from build123d import *

# Parameters (mm, degrees)
CUT_EXTRUDE1_DEPTH      = 10
BOSS_EXTRUDE1_DEPTH     = 30
CUT_EXTRUDE2_DEPTH      = 752.943114111524
CUT_EXTRUDE2_DEPTH_BACK = 752.943114111524
SKETCH5_R               = 4.999999999999998
SKETCH6_R               = 40.00000000000003
CUT_EXTRUDE3_DEPTH      = 752.943114111524
BOSS_EXTRUDE3_DEPTH     = 5
CUT_EXTRUDE4_DEPTH      = 752.943114111524
CUT_EXTRUDE4_DEPTH_BACK = 752.943114111524
FILLET1_R               = 5
FILLET2_R               = 4.5
CUT_EXTRUDE5_REACH      = 769.798
SKETCH13_R              = 4.999999999999991
CUT_EXTRUDE6_REACH      = 787.596
SKETCH14_R              = 4.999999999999991
SKETCH14_R_2            = 4.999999999999939


with BuildPart() as part:
    # Sweep2: sweep along a path in Sketch1
    with BuildLine(Plane.XY) as sweep2_path:
        Line((0, 0), (379.6, 0))
        ThreePointArc((379.6, 0), (450.3106781186548, -29.289321881345245), (479.6, -99.99999999999997))
        Line((479.6, -99.99999999999997), (479.6, -360))
        ThreePointArc((479.6, -360), (470.81320343559645, -381.21320343559637), (449.6000000000001, -390))
        Line((449.6000000000001, -390), (370.00000000000006, -390))
    # Sketch2 → Sweep2 (sweep)
    with BuildSketch(Plane(origin=(0, 0, 0), x_dir=(0, 0, -1), z_dir=(1, 0, 0))):
        with BuildLine():
            Line((-360.49999999999994, 27.89826377546352), (360.50000000000006, 27.89826377546352))
            ThreePointArc((360.50000000000006, 27.89826377546352), (363.68198051533955, 26.580244290802984), (365.00000000000006, 23.39826377546352))
            Line((365.00000000000006, 23.39826377546352), (365.00000000000006, 22.89826377546352))
            Line((365.00000000000006, 22.89826377546352), (-364.99999999999994, 22.89826377546352))
            Line((-364.99999999999994, 22.89826377546352), (-364.99999999999994, 23.39826377546352))
            ThreePointArc((-364.99999999999994, 23.39826377546352), (-363.68198051533943, 26.580244290802984), (-360.49999999999994, 27.89826377546352))
        make_face()
    sweep(path=sweep2_path.line)

    # Sketch3 → Cut-Extrude1 (cut)
    with BuildSketch(Plane(origin=(0, 27.89826377546352, 0), x_dir=(1, 0, 0), z_dir=(0, 1, 0))):
        Polygon((-8.83e-15, 60), (30.00000000000002, 60), (30.00000000000002, 90.00000000000003), (-6.99e-15, 90.00000000000003), align=None)
        Polygon((-8.83e-15, -60), (30.00000000000002, -60), (30.00000000000002, -90.00000000000003), (-6.99e-15, -90.00000000000003), align=None)
    extrude(amount=-CUT_EXTRUDE1_DEPTH, mode=Mode.SUBTRACT)

    # Sketch4 → Boss-Extrude1 (add)
    with BuildSketch(Plane(origin=(0, 27.89826377546352, 0), x_dir=(1, 0, 0), z_dir=(0, 1, 0))):
        Polygon((0, -90.00000000000003), (30.00000000000002, -90.00000000000003), (30.00000000000002, -95.00000000000003), (6.1e-16, -95.00000000000003), align=None)
        Polygon((-8.83e-15, -60), (30.00000000000002, -60), (30.00000000000002, -54.99999999999999), (0, -54.99999999999999), align=None)
        Polygon((6.1e-16, 95.00000000000003), (30.00000000000002, 95.00000000000003), (30.00000000000002, 90.00000000000003), (0, 90.00000000000003), align=None)
        Polygon((0, 54.99999999999999), (30.00000000000002, 54.99999999999999), (30.00000000000002, 60), (-8.83e-15, 60), align=None)
    extrude(amount=BOSS_EXTRUDE1_DEPTH)

    # Sketch5 → Cut-Extrude2 (cut, two sides: drawn at the far end of the back side and taken through both)
    with BuildSketch(Plane.XY.offset(-CUT_EXTRUDE2_DEPTH_BACK)):
        with Locations((15.000000000000012, 42.89826377546352)):
            Circle(SKETCH5_R)
    extrude(amount=CUT_EXTRUDE2_DEPTH + CUT_EXTRUDE2_DEPTH_BACK, mode=Mode.SUBTRACT)

    # Sketch6 → Cut-Extrude3 (cut, through all)
    with BuildSketch(Plane(origin=(0, 0, 0), x_dir=(0, 0, -1), z_dir=(1, 0, 0))):
        with Locations(Location((-104.49999999999999, -85.90173622453648, 0), (0, 0, 200.637645216))):
            Circle(SKETCH6_R)
        with Locations(Location((25.50000000000002, -85.90173622453648, 0), (0, 0, 200.637645216))):
            Circle(SKETCH6_R)
    extrude(amount=CUT_EXTRUDE3_DEPTH, mode=Mode.SUBTRACT)

    # Sketch9 → Boss-Extrude3 (add)
    with BuildSketch(Plane(origin=(0, 0, -365.00000000000006), x_dir=(-1, 0, 0), z_dir=(0, 0, -1))):
        with BuildLine():
            Line((0, 22.898263775463516), (-379.6, 22.898263775463516))
            ThreePointArc((-379.6, 22.898263775463516), (-466.50219571168327, -13.097804288316723), (-502.49826377546356, -99.99999999999997))
            Line((-502.49826377546356, -99.99999999999997), (-502.49826377546356, -360))
            ThreePointArc((-502.49826377546356, -360), (-487.0047210286247, -397.4047210286247), (-449.6000000000001, -412.89826377546353))
            Line((-449.6000000000001, -412.89826377546353), (-370.00000000000006, -412.89826377546353))
            Line((-370.00000000000006, -412.89826377546353), (-370.00000000000006, -417.89826377546353))
            Line((-370.00000000000006, -417.89826377546353), (0, -417.89826377546353))
            Line((0, -417.89826377546353), (0, -412.89826377546353))
            Line((0, -412.89826377546353), (0, 22.898263775463516))
        make_face()
    boss_extrude3 = extrude(amount=-BOSS_EXTRUDE3_DEPTH)

    # Mirror3: Boss-Extrude3 across plane
    add(boss_extrude3.mirror(Plane.XY))

    # Sketch11 → Cut-Extrude4 (cut, two sides: drawn at the far end of the back side and taken through both)
    with BuildSketch(Plane.XY.offset(-CUT_EXTRUDE4_DEPTH_BACK)):
        with BuildLine():
            Line((149.99826377546347, -297.89826377546353), (149.99826377546347, -397.89826377546353))
            ThreePointArc((149.99826377546347, -397.89826377546353), (152.927195963598, -404.969331587329), (159.99826377546347, -407.8982637754636))
            Line((159.99826377546347, -407.8982637754636), (239.99826377546347, -407.8982637754636))
            ThreePointArc((239.99826377546347, -407.8982637754636), (247.06933158732897, -404.96933158732907), (249.99826377546347, -397.89826377546353))
            Line((249.99826377546347, -397.89826377546353), (249.99826377546347, -297.89826377546353))
            ThreePointArc((249.99826377546347, -297.89826377546353), (199.99826377546347, -247.89826377546353), (149.99826377546347, -297.89826377546353))
        make_face()
    extrude(amount=CUT_EXTRUDE4_DEPTH + CUT_EXTRUDE4_DEPTH_BACK, mode=Mode.SUBTRACT)

    # Fillet1
    fillet1_edges = [part.edges().sort_by_distance(p)[0] for p in [
        (247.06933158732897, -404.96933158732907, -365.00000000000006),
        (247.06933158732897, -404.96933158732907, 364.99999999999994),
        (199.99826377546344, -407.8982637754636, -365.00000000000006),
        (199.99826377546344, -407.8982637754636, 364.99999999999994),
        (152.927195963598, -404.969331587329, -365.00000000000006),
        (152.927195963598, -404.969331587329, 364.99999999999994),
        (149.99826377546347, -347.89826377546353, -365.00000000000006),
        (149.99826377546347, -347.89826377546353, 364.99999999999994),
        (199.99826377546347, -247.89826377546353, -365.00000000000006),
        (199.99826377546347, -247.89826377546353, 364.99999999999994),
        (249.99826377546347, -347.89826377546353, -365.00000000000006),
        (249.99826377546347, -347.89826377546353, 364.99999999999994),
    ]]
    fillet(fillet1_edges, radius=FILLET1_R - 0.0001)  # a hair under: the kernel refuses the full size

    # Fillet2
    fillet2_edges = [part.edges().sort_by_distance(p)[0] for p in [
        (185.00000000000003, -417.89826377546353, -365.00000000000006),
        (185.00000000000003, -417.89826377546353, 365.00000000000006),
    ]]
    fillet(fillet2_edges, radius=FILLET2_R)

    # Sketch13 → Cut-Extrude5 (cut, up to next)
    with BuildSketch(Plane(origin=(0, 27.89826377546352, 0), x_dir=(1, 0, 0), z_dir=(0, 1, 0)), mode=Mode.PRIVATE) as cut_extrude5_sk1:
        with Locations(Location((176.31641992134345, -229.13071131685336, 0), (0, 0, 270))):
            Circle(SKETCH13_R)
    cut_extrude5_tool1 = extrude(cut_extrude5_sk1.sketch, amount=-CUT_EXTRUDE5_REACH, mode=Mode.PRIVATE) & part.part
    # Sketch13 → Cut-Extrude5 (cut, up to next)
    with BuildSketch(Plane(origin=(0, 27.89826377546352, 0), x_dir=(1, 0, 0), z_dir=(0, 1, 0)), mode=Mode.PRIVATE) as cut_extrude5_sk2:
        with Locations(Location((277.4164199213434, -295.869288683147, 0), (0, 0, 270))):
            Circle(SKETCH13_R)
    cut_extrude5_tool2 = extrude(cut_extrude5_sk2.sketch, amount=-CUT_EXTRUDE5_REACH, mode=Mode.PRIVATE) & part.part
    # Sketch13 → Cut-Extrude5 (cut, up to next)
    with BuildSketch(Plane(origin=(0, 27.89826377546352, 0), x_dir=(1, 0, 0), z_dir=(0, 1, 0)), mode=Mode.PRIVATE) as cut_extrude5_sk3:
        with Locations(Location((277.4164199213434, -229.13071131685336, 0), (0, 0, 270))):
            Circle(SKETCH13_R)
    cut_extrude5_tool3 = extrude(cut_extrude5_sk3.sketch, amount=-CUT_EXTRUDE5_REACH, mode=Mode.PRIVATE) & part.part
    # Sketch13 → Cut-Extrude5 (cut, up to next)
    with BuildSketch(Plane(origin=(0, 27.89826377546352, 0), x_dir=(1, 0, 0), z_dir=(0, 1, 0)), mode=Mode.PRIVATE) as cut_extrude5_sk4:
        with Locations(Location((176.31641992134345, -295.869288683147, 0), (0, 0, 270))):
            Circle(SKETCH13_R)
    cut_extrude5_tool4 = extrude(cut_extrude5_sk4.sketch, amount=-CUT_EXTRUDE5_REACH, mode=Mode.PRIVATE) & part.part
    # Sketch13 → Cut-Extrude5 (cut, up to next)
    with BuildSketch(Plane(origin=(0, 27.89826377546352, 0), x_dir=(1, 0, 0), z_dir=(0, 1, 0)), mode=Mode.PRIVATE) as cut_extrude5_sk5:
        with Locations(Location((277.4164199213434, 229.13071131685336, 0), (0, 0, 270))):
            Circle(SKETCH13_R)
    cut_extrude5_tool5 = extrude(cut_extrude5_sk5.sketch, amount=-CUT_EXTRUDE5_REACH, mode=Mode.PRIVATE) & part.part
    # Sketch13 → Cut-Extrude5 (cut, up to next)
    with BuildSketch(Plane(origin=(0, 27.89826377546352, 0), x_dir=(1, 0, 0), z_dir=(0, 1, 0)), mode=Mode.PRIVATE) as cut_extrude5_sk6:
        with Locations(Location((176.31641992134345, 229.13071131685336, 0), (0, 0, 270))):
            Circle(SKETCH13_R)
    cut_extrude5_tool6 = extrude(cut_extrude5_sk6.sketch, amount=-CUT_EXTRUDE5_REACH, mode=Mode.PRIVATE) & part.part
    # Sketch13 → Cut-Extrude5 (cut, up to next)
    with BuildSketch(Plane(origin=(0, 27.89826377546352, 0), x_dir=(1, 0, 0), z_dir=(0, 1, 0)), mode=Mode.PRIVATE) as cut_extrude5_sk7:
        with Locations(Location((176.31641992134345, 295.869288683147, 0), (0, 0, 270))):
            Circle(SKETCH13_R)
    cut_extrude5_tool7 = extrude(cut_extrude5_sk7.sketch, amount=-CUT_EXTRUDE5_REACH, mode=Mode.PRIVATE) & part.part
    # Sketch13 → Cut-Extrude5 (cut, up to next)
    with BuildSketch(Plane(origin=(0, 27.89826377546352, 0), x_dir=(1, 0, 0), z_dir=(0, 1, 0)), mode=Mode.PRIVATE) as cut_extrude5_sk8:
        with Locations(Location((277.4164199213434, 295.869288683147, 0), (0, 0, 270))):
            Circle(SKETCH13_R)
    cut_extrude5_tool8 = extrude(cut_extrude5_sk8.sketch, amount=-CUT_EXTRUDE5_REACH, mode=Mode.PRIVATE) & part.part
    add(cut_extrude5_tool1.solids().sort_by_distance((176.31642, 27.898264, 229.130711))[0], mode=Mode.SUBTRACT)
    add(cut_extrude5_tool2.solids().sort_by_distance((277.41642, 27.898264, 295.869289))[0], mode=Mode.SUBTRACT)
    add(cut_extrude5_tool3.solids().sort_by_distance((277.41642, 27.898264, 229.130711))[0], mode=Mode.SUBTRACT)
    add(cut_extrude5_tool4.solids().sort_by_distance((176.31642, 27.898264, 295.869289))[0], mode=Mode.SUBTRACT)
    add(cut_extrude5_tool5.solids().sort_by_distance((277.41642, 27.898264, -229.130711))[0], mode=Mode.SUBTRACT)
    add(cut_extrude5_tool6.solids().sort_by_distance((176.31642, 27.898264, -229.130711))[0], mode=Mode.SUBTRACT)
    add(cut_extrude5_tool7.solids().sort_by_distance((176.31642, 27.898264, -295.869289))[0], mode=Mode.SUBTRACT)
    add(cut_extrude5_tool8.solids().sort_by_distance((277.41642, 27.898264, -295.869289))[0], mode=Mode.SUBTRACT)

    # Sketch14 → Cut-Extrude6 (cut, up to next)
    with BuildSketch(Plane.XZ.offset(417.89826377546353), mode=Mode.PRIVATE) as cut_extrude6_sk1:
        with Locations(Location((390.00000000000006, 99.99999999999999, 0), (0, 0, 270))):
            Circle(SKETCH14_R)
    cut_extrude6_tool1 = extrude(cut_extrude6_sk1.sketch, amount=-CUT_EXTRUDE6_REACH, mode=Mode.PRIVATE) & part.part
    # Sketch14 → Cut-Extrude6 (cut, up to next)
    with BuildSketch(Plane.XZ.offset(417.89826377546353), mode=Mode.PRIVATE) as cut_extrude6_sk2:
        with Locations(Location((390.0000000000002, -100.00000000000018, 0), (0, 0, 90))):
            Circle(SKETCH14_R_2)
    cut_extrude6_tool2 = extrude(cut_extrude6_sk2.sketch, amount=-CUT_EXTRUDE6_REACH, mode=Mode.PRIVATE) & part.part
    add(cut_extrude6_tool1.solids().sort_by_distance((390, -417.898264, 100))[0], mode=Mode.SUBTRACT)
    add(cut_extrude6_tool2.solids().sort_by_distance((390, -417.898264, -100))[0], mode=Mode.SUBTRACT)


solid = part.part
Verification items for the finished model (mm, model axes). A direction names the side the tool comes from. Round coordinates to 2 decimals unless told otherwise and drop trailing zeros. Loops run counter-clockwise (first coordinate to the right, second up) from the corner with the lowest first, then second, coordinate; pieces in that order, holes last. Notation, with made-up numbers: (3, 6.25) - (37, 6.25) arc R8 ccw to (37, 19.25) - close; hole circle Ø4 at (-38.5, 41). An arc over 180 degrees is marked (long way). Write item = value, one per line.
Q1. Mould release check, pull along Z, two halves, no side actions. Record for faces 1 (the cylindrical face through (501.28, -67.82, 10.18)), 2 (the cylindrical face through (490.988, -400.488, 5.047)), 3 (the flat face through (255, -192, -365)), 4 (the flat face through (255, -192, 365)): +Z half, -Z half, draft (parallel to the pull), parting line (faces both ways), or undercut.
Here are the results:
face_1 = undercut
face_2 = draft
face_3 = -Z half
face_4 = +Z half
Q2. Sectioned sample at D-D on y = -89. State how many separate pieces and enclosed holes the cut face has, plus the area to 3 significant figures.
Here are the results:
separate_pieces = 3
enclosed_holes = 0
area = 7,870 mm^2
Q3. Sectioned sample at A-A on z = -25.5. Record the boundary of the cut face in (x, y).
Here are the results:
outline = (0, 22.9) - (379.6, 22.9) arc R122.9 cw to (489.95, -45.9) - (495.49, -45.9) arc R127.9 ccw to (379.6, 27.9) - (0, 27.9) - close; (370, -417.9) - (449.6, -417.9) arc R57.9 ccw to (507.5, -360) - (507.5, -125.9) - (502.5, -125.9) - (502.5, -360) arc R52.9 cw to (449.6, -412.9) - (370, -412.9) - close
Q4. Sectioned sample at B-B on y = -142. Record the boundary of the cut face in (x, z), plus the area to 3 significant figures.
Here are the results:
outline = (0, -365) - (503, -365) arc R4.5 ccw to (507.5, -360.5) - (507.5, 360.5) arc R4.5 ccw to (503, 365) - (0, 365) - (0, 360) - (502.5, 360) - (502.5, -360) - (0, -360) - close
area = 8,670 mm^2
Q5. Depth check by flat-ended pin: pin 1 (1.5 mm diameter, centred on y = -58, z = -273.5, fed in from -X); pin 2 (13 mm diameter, centred on x = 176.32, z = -229.13, fed in from -Y); pin 3 (9 mm diameter, centred on x = 277.42, z = -229.13, fed in from +Y); pin 4 (1.5 mm diameter, centred on y = 49, z = 92, fed in from +X). Enter the tip coordinate at first touch or a pass-through.
Here are the results:
pin_1 = 494.82
pin_2 = 22.9
pin_3 = through
pin_4 = 30
Q6. Tool access check on faces 5 (the flat face through (15, 37, -60)), 6 (the cylindrical face through (487.414, -396.991, -5.04)), 7 (the flat face through (11, 39, -55)). Record the directions out of +Z, -Z, +X, -X, +Y, -Y that give a thin tool (end or side, any length) a straight path to the whole face; none if there is none.
Here are the results:
face_5 = -X, +Y, -Y
face_6 = -X
face_7 = +X, -X, +Y
Q7. Sectioned sample at C-C on z = -279. Record the boundary of the cut face in (x, y).
Here are the results:
outline = (0, 22.9) - (379.6, 22.9) arc R122.9 cw to (502.5, -100) - (502.5, -360) arc R52.9 cw to (449.6, -412.9) - (370, -412.9) - (370, -417.9) - (449.6, -417.9) arc R57.9 ccw to (507.5, -360) - (507.5, -100) arc R127.9 ccw to (379.6, 27.9) - (0, 27.9) - close
Q8. Material ranges on L1, parallel to Z at x = 410, y = -155; L2, parallel to Y at x = 253, z = -116.5; L3, parallel to Y at x = 15, z = 57, recorded low to high.
Here are the results:
L1 = -365 to -360, 360 to 365
L2 = 22.9 to 27.9
L3 = 22.9 to 37.9, 47.9 to 57.9
